Build history of the part. All positions in model axes, mm. Give positions to 0.01 mm unless a question says otherwise; leave off trailing zeros. Write each loop counter-clockwise with the first axis right and the second up, starting at its lowest first coordinate (ties: lowest second). Pieces come first, ordered by that corner, then holes. Notation, with made-up numbers: M 12.25,36.25 L 50.25,36.25 A25 ccw 50.25,74.25 Z; hole C 20,33.25 d7. An arc over 180 degrees is marked long. One line per item, written item: value. Start each with the question number.
from build123d import *

# Parameters (mm, degrees)
SKIZZE1_W                       = 15
SKIZZE1_H                       = 5.9
AUFSATZ_LINEAR_AUSTRAGEN1_DEPTH = 20
SCHNITT_LINEAR_AUSTRAGEN1_DEPTH = 6.4
SCHNITT_LINEAR_AUSTRAGEN2_DEPTH = 6.4
SKIZZE4_W                       = 1.6
SKIZZE4_H                       = 7.2
AUFSATZ_LINEAR_AUSTRAGEN2_DEPTH = 2


with BuildPart() as part:
    # Skizze1 → Aufsatz-Linear austragen1 (new body)
    with BuildSketch(Plane(origin=(0, 0, 0), x_dir=(1, 0, 0), z_dir=(0, 1, 0))):
        Polygon((20, -5.9), (0, -5.9), (0, -15.9), (10, -15.9), align=None)
        Polygon((0, -5.9), (0, -15.9), (-15, -5.9), align=None)
        with Locations((-7.5, -2.95)):
            Rectangle(SKIZZE1_W, SKIZZE1_H)
        Polygon((0, 10), (0, 0), (-15, 0), align=None)
        Polygon((0, 10), (0, 0), (80, 0), (80, 10), (70, 10), align=None)
        Polygon((80, 10), (80, 0), (220, 0), (216.360297657, 10), (112, 10), align=None)
        Polygon((80, 20), (80, 10), (112, 10), (102, 20), align=None)
        Polygon((70, 10), (80, 10), (80, 20), align=None)
    extrude(amount=AUFSATZ_LINEAR_AUSTRAGEN1_DEPTH)

    # Skizze2 → Schnitt-Linear austragen1 (cut)
    with BuildSketch(Plane(origin=(0, 20, 0), x_dir=(1, 0, 0), z_dir=(0, 1, 0))):
        Polygon((70, 10), (112, 10), (102, 20), (80, 20), align=None)
    extrude(amount=-SCHNITT_LINEAR_AUSTRAGEN1_DEPTH, mode=Mode.SUBTRACT)

    # Skizze3 → Schnitt-Linear austragen2 (cut)
    with BuildSketch(Plane.XZ):
        Polygon((70, -10), (112, -10), (102, -20), (80, -20), align=None)
    extrude(amount=-SCHNITT_LINEAR_AUSTRAGEN2_DEPTH, mode=Mode.SUBTRACT)

    # Skizze4 → Aufsatz-Linear austragen2 (add)
    with BuildSketch(Plane(origin=(0, 0, -20), x_dir=(-1, 0, 0), z_dir=(0, 0, -1))):
        with Locations((-101.2, 10)):
            Rectangle(SKIZZE4_W, SKIZZE4_H)
    extrude(amount=AUFSATZ_LINEAR_AUSTRAGEN2_DEPTH)


solid = part.part
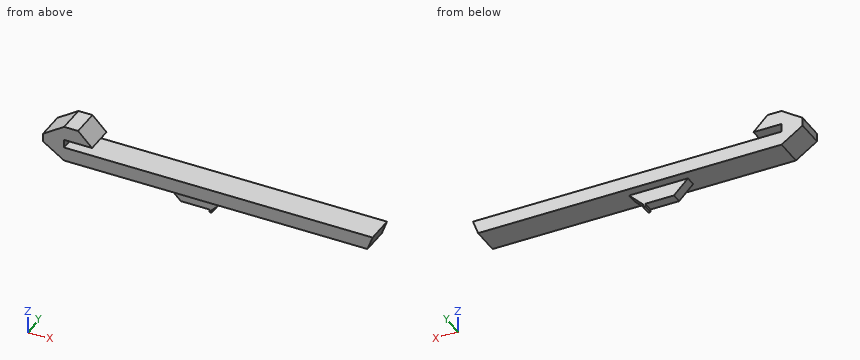
1) Drop flat-ended pins along their axis: P1, Ø1, axis at y = 10, z = -21, coming from the -X side; P2, Ø1.5, axis at y = 8, z = -17, coming from the -X side; P3, Ø3, axis at y = 9.5, z = -15.5, coming from the +X side. Give the stop position or say it passes through.
2) Band-saw the part on C-C (x = 134.5). List the corners of the cut face in (y, z).
3) Band-saw the part on B-B (z = -13). List the corners of the cut face in (x, y).
4) Band-saw the part on A-A (y = 11.5). List the corners of the cut face in (x, z).
5) Probe line 1 along Z through (x, y) = (10, 4.5); line 2 along Z through (x, y) = (158, 4.5); line 3 along Y through (x, z) = (77, -14). List the from-to ranges inside material, lowest first. Write a range as from..to.
Model answer:
1. P1: stops at x = 100.4
1. P2: stops at x = 76.25
1. P3: stops at x = 108
2. outline: M 0,-10 L 20,-10 L 20,0 L 0,0 Z
3. outline: M 73,6.4 L 109,6.4 L 109,13.6 L 73,13.6 Z
4. outline: M -15,0 L 0,-10 L 70,-10 L 80,-20 L 100.4,-20 L 100.4,-22 L 102,-22 L 102,-20 L 112,-10 L 216.36,-10 L 220,0 L 0,0 L 0,5.9 L 20,5.9 L 10,15.9 L 0,15.9 L -15,5.9 Z
5. line 1: z = -10..0, 5.9..15.9
5. line 2: z = -10..0
5. line 3: y = 6.4..13.6
